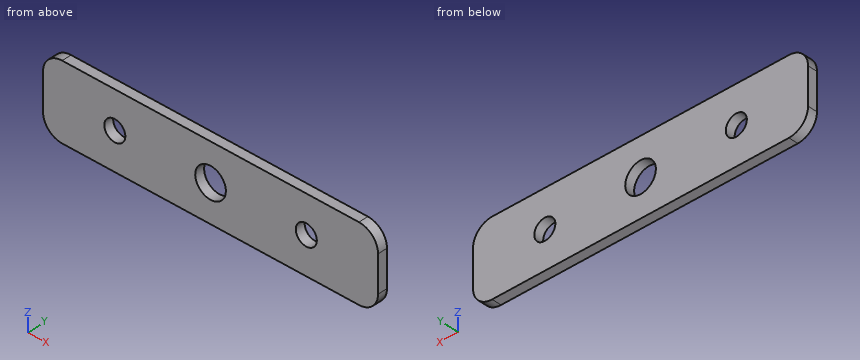
```python
from build123d import *

# Parameters (mm, degrees)
CROQUIS1_W                 = 70
CROQUIS1_H                 = 15.6
SALIENTE_EXTRUIR1_DEPTH    = 2
CORTAR_EXTRUIR2_DEPTH      = 36.914342539
CORTAR_EXTRUIR2_DEPTH_BACK = 36.914342539
CROQUIS3_R                 = 3.2
CROQUIS3_R_2               = 2.2
REDONDEO1_R                = 4


with BuildPart() as part:
    # Croquis1 → Saliente-Extruir1 (new body)
    with BuildSketch(Plane(origin=(0, 0, 0), x_dir=(1, 0, 0), z_dir=(0, 1, 0))):
        Rectangle(CROQUIS1_W, CROQUIS1_H)
    extrude(amount=SALIENTE_EXTRUIR1_DEPTH)

    # Croquis3 → Cortar-Extruir2 (cut, two sides: drawn at the far end of the back side and taken through both)
    with BuildSketch(Plane(origin=(0, 0, 0), x_dir=(1, 0, 0), z_dir=(0, 1, 0)).offset(-CORTAR_EXTRUIR2_DEPTH_BACK)):
        with Locations(Location((0, 0, 0), (0, 0, 90))):
            Circle(CROQUIS3_R)
        with Locations(Location((20, 0, 0), (0, 0, 90))):
            Circle(CROQUIS3_R_2)
        with Locations(Location((-20, 0, 0), (0, 0, 90))):
            Circle(CROQUIS3_R_2)
    extrude(amount=CORTAR_EXTRUIR2_DEPTH + CORTAR_EXTRUIR2_DEPTH_BACK, mode=Mode.SUBTRACT)

    # Redondeo1
    redondeo1_edges = [part.edges().sort_by_distance(p)[0] for p in [
        (35, 1, 7.8),
        (-35, 1, 7.8),
        (-35, 1, -7.8),
        (35, 1, -7.8),
    ]]
    fillet(redondeo1_edges, radius=REDONDEO1_R)


solid = part.part
```
Input: part model. Units: mm. Frame: model coordinates. Give positions to 0.01 mm unless a question says otherwise; leave off trailing zeros. Order: outer loops, then holes, each group sorted by start corner. A loop starts at its lowest first (then second) coordinate and runs counter-clockwise, first axis right, second up. Notation, with made-up numbers: (-23.75, 73) - (28.25, 73) arc R19 cw to (28.25, 100) - close; hole circle Ø11 at (83.5, -6.5). An arc over 180 degrees is marked (long way). Use a Markdown table: item, result.
(1) Section query B-B (y = 0.9). Output: boundary loops of the cut face in (x, z).
Computed values:
| item | result |
|---|---|
| outline | (-35, -3.8) arc R4 ccw to (-31, -7.8) - (31, -7.8) arc R4 ccw to (35, -3.8) - (35, 3.8) arc R4 ccw to (31, 7.8) - (-31, 7.8) arc R4 ccw to (-35, 3.8) - close; hole circle Ø4.4 at (-20, 0); hole circle Ø6.4 at (0, 0); hole circle Ø4.4 at (20, 0) |
(2) Section query D-D (x = 20). Output: boundary loops of the cut face in (y, z), then the cut area to 3 significant figures.
Computed values:
| item | result |
|---|---|
| outline | (0, -7.8) - (2, -7.8) - (2, -2.2) - (0, -2.2) - close; (0, 2.2) - (2, 2.2) - (2, 7.8) - (0, 7.8) - close |
| area | 22.4 mm2 |
(3) Section query C-C (z = 0). Output: boundary loops of the cut face in (x, y), then the cut area to 3 significant figures.
Computed values:
| item | result |
|---|---|
| outline | (-35, 0) - (-22.2, 0) - (-22.2, 2) - (-35, 2) - close; (-17.8, 0) - (-3.2, 0) - (-3.2, 2) - (-17.8, 2) - close; (3.2, 0) - (17.8, 0) - (17.8, 2) - (3.2, 2) - close; (22.2, 0) - (35, 0) - (35, 2) - (22.2, 2) - close |
| area | 110 mm2 |
(4) Section query A-A (x = 0). Output: boundary loops of the cut face in (y, z), then the cut area to 3 significant figures.
Computed values:
| item | result |
|---|---|
| outline | (0, -7.8) - (2, -7.8) - (2, -3.2) - (0, -3.2) - close; (0, 3.2) - (2, 3.2) - (2, 7.8) - (0, 7.8) - close |
| area | 18.4 mm2 |
(5) Line query: line 1 (X direction, y = 0.55, z = 0); line 2 (X direction, y = 0.35, z = 0.5); line 3 (X direction, y = 0.45, z = -4) (3 decimals). Output: solid intervals per line, ascending. Write a range as from..to.
Computed values:
| item | result |
|---|---|
| line 1 | x = -35..-22.2, -17.8..-3.2, 3.2..17.8, 22.2..35 |
| line 2 | x = -35..-22.14, -17.86..-3.16, 3.16..17.86, 22.14..35 |
| line 3 | x = -34.995..34.995 |
